```python
from build123d import *

# Parameters (mm, degrees)
SKETCH1_R           = 3.5
SKETCH1_R_2         = 2.63
SKETCH1_R_3         = 1.6
BOSS_EXTRUDE1_DEPTH = 17
SKETCH2_R           = 4.675
BOSS_EXTRUDE2_DEPTH = 2.31
CUT_EXTRUDE1_DEPTH  = 18.975139222
BOSS_EXTRUDE3_START = 17
SKETCH1_3_R         = 3.5
SKETCH1_3_R_2       = 2.63
BOSS_EXTRUDE3_DEPTH = 3
SKETCH5_R           = 1.535
CUT_EXTRUDE2_DEPTH  = 23.152779282
CHAMFER1_SIZE       = 1


with BuildPart() as part:
    # Sketch1 → Boss-Extrude1 (new body)
    # profile 1 of 2: a face of its own
    with BuildSketch(Plane(origin=(0, 0, 0), x_dir=(0, 0, -1), z_dir=(1, 0, 0))):
        Circle(SKETCH1_R)
        Circle(SKETCH1_R_2, mode=Mode.SUBTRACT)
    # profile 2 of 2: a face of its own
    with BuildSketch(Plane(origin=(0, 0, 0), x_dir=(0, 0, -1), z_dir=(1, 0, 0))):
        Circle(SKETCH1_R_2)
        Circle(SKETCH1_R_3, mode=Mode.SUBTRACT)
    extrude(amount=BOSS_EXTRUDE1_DEPTH)

    # Sketch2 → Boss-Extrude2 (add, symmetric)
    with BuildSketch(Plane(origin=(0, 0, 0), x_dir=(1, 0, 0), z_dir=(0, 1, 0))):
        Circle(SKETCH2_R)
    extrude(amount=BOSS_EXTRUDE2_DEPTH, both=True)

    # Sketch3 → Cut-Extrude1 (cut, symmetric)
    with BuildSketch(Plane.XY):
        Polygon((66.444481418, 11.326116973), (12.125, 3.5), (3.865452755, 2.31), (-4.675, 2.31), (-59.55536232, 2.31), (-67.389432633, 111.790792909), (58.610411105, 120.806909882), align=None)
    cut_extrude1 = extrude(amount=CUT_EXTRUDE1_DEPTH, both=True, mode=Mode.SUBTRACT)

    # Mirror1: Cut-Extrude1 across plane
    add(cut_extrude1.mirror(Plane.ZX), mode=Mode.SUBTRACT)

    # Sketch1<3> → Boss-Extrude3 (add)
    with BuildSketch(Plane(origin=(0, 0, 0), x_dir=(0, 0, -1), z_dir=(1, 0, 0)).offset(BOSS_EXTRUDE3_START)):
        with Locations(Location((0, 0, 0), (0, 0, 221.299872792))):
            Circle(SKETCH1_3_R)
        Circle(SKETCH1_3_R_2, mode=Mode.SUBTRACT)
    extrude(amount=BOSS_EXTRUDE3_DEPTH)

    # Sketch4 → Revolve1 (revolve)
    with BuildSketch(Plane.XY, mode=Mode.PRIVATE) as revolve1_sk:
        Polygon((0, 4.15), (2.65, 4.15), (2.65, 3.95), (1.94, 3.24), (1.94, 2.31), (0, 2.31), align=None)
    revolve1 = revolve(revolve1_sk.sketch.rotate(Axis((0, 2.31, 0), (0, 1, 0)), 90), axis=Axis((0, 2.31, 0), (0, 1, 0)))

    # Mirror2: Revolve1 across plane
    add(revolve1.mirror(Plane.ZX))

    # Sketch5 → Cut-Extrude2 (cut, through all)
    with BuildSketch(Plane(origin=(0, 4.15, 0), x_dir=(1, 0, 0), z_dir=(0, 1, 0))):
        with Locations(Location((0, 0, 0), (0, 0, 270))):
            Circle(SKETCH5_R)
    extrude(amount=-CUT_EXTRUDE2_DEPTH, mode=Mode.SUBTRACT)

    # Chamfer1
    chamfer1_edges = [part.edges().sort_by_distance(p)[0] for p in [
        (17, 0, 2.63),
    ]]
    chamfer(chamfer1_edges, length=CHAMFER1_SIZE)


solid = part.part
```
Could you check a few things on this model? Use its own coordinates, in mm. A direction names the side the tool comes from. Give positions to 0.01 mm unless a question says otherwise; leave off trailing zeros. Order: outer loops, then holes, each group sorted by start corner. A loop starts at its lowest first (then second) coordinate and runs counter-clockwise, first axis right, second up.
Q1. For faces 5 (the flat face through (7.14, -2.78, 0.04)), 6 (the cylindrical face through (-0.58, 2.77, -1.85)), 7 (the flat face through (0, -4.15, 2)), which set-ups out of +Z, -Z, +X, -X, +Y, -Y let a thin tool reach every point of the face, with its end or its side?
Q2. Suppose I cut it at B-B, the plane y = 0. Write out the boundary of the cut face in (x, z) (3 decimals).
Q3. Suppose I cut it at C-C, the plane z = 2.25. Count the separate pieces of the cut face and the enclosed holes in it, and give its area (3 significant figures).
Q4. Suppose I cut it at A-A, the plane x = 0. Write out the boundary of the cut face in (y, z) (3 decimals).
Q5. We'd pull the mould along X, two halves only. Please class faces 1 (the flat face through (20, -3, -1)), 2 (the flat face through (7.14, 2.78, 0.04)), 3 (the cylindrical face through (-4.67, 0.03, -0.17)), 4 (the cylindrical face through (10.61, -0.97, 1.27)): +X half, -X half, draft (parallel to the pull), parting line (faces both ways), or undercut.
Q6. If I drill on line 1 along Y through (x, z) = (18.65, 0); line 2 along X through (y, z) = (0, 1); line 3 along Y through (x, z) = (11, 0), over which ranges is the centre line in solid material (lowest first)?
Q7. Suppose I cut it at D-D, the plane x = 8.5. Write out the boundary of the cut face in (y, z), and give its area (3 significant figures).
Q8. I'm going to push flat-ended pins straight in: P1, Ø1.5, axis at x = 13.5, y = 1.5, coming from the -Z side; P2, Ø4, axis at y = -2.5, z = -3.5, coming from the -X side; P3, Ø1, axis at y = -1.5, z = -3, coming from the -X side; P4, Ø3, axis at x = 0, z = 0, coming from the +Y side. Where does each tip first touch, or does it pass through?
Solution:
1. face 5: +Z, -Z, -Y
1. face 6: none
1. face 7: +Z, -Z, +X, -X, -Y
2. outline: (3.099, -3.5) - (20, -3.5) - (20, -2.63) - (18, -2.63) - (17, -1.63) - (17, -1.6) - (4.393, -1.6) arc R4.675 ccw to (4.393, 1.6) - (17, 1.6) - (17, 1.63) - (18, 2.63) - (20, 2.63) - (20, 3.5) - (3.099, 3.5) arc R4.675 ccw (long way) to start; hole circle Ø3.07 at (0, 0)
3. separate pieces: 3
3. enclosed holes: 0
3. area: 119 mm2
4. outline: (-4.15, -2.65) - (-3.95, -2.65) - (-3.24, -1.94) - (-2.31, -1.94) - (-2.31, -4.675) - (2.31, -4.675) - (2.31, -1.94) - (3.24, -1.94) - (3.95, -2.65) - (4.15, -2.65) - (4.15, -1.535) - (-4.15, -1.535) - close; (-4.15, 1.535) - (4.15, 1.535) - (4.15, 2.65) - (3.95, 2.65) - (3.24, 1.94) - (2.31, 1.94) - (2.31, 4.675) - (-2.31, 4.675) - (-2.31, 1.94) - (-3.24, 1.94) - (-3.95, 2.65) - (-4.15, 2.65) - close
5. face 1: +X half
5. face 2: undercut
5. face 3: parting line
5. face 4: draft
6. line 1: y = -3.5 to -2.63, 2.63 to 3.5
6. line 2: x = -4.57 to -1.16, 1.16 to 4.57
6. line 3: y = -3.34 to -1.6, 1.6 to 3.34
7. outline: (-2.98, -1.84) arc R3.5 ccw to (2.98, -1.84) - (2.98, 1.84) arc R3.5 ccw to (-2.98, 1.84) - close; hole circle Ø3.2 at (0, 0)
7. area: 27.8 mm2
8. P1: stops at z = -3.42
8. P2: stops at x = -4.42
8. P3: stops at x = -3.95
8. P4: passes through
